The model under review builds one solid part; all positions refer to its coordinate system, in mm. A direction names the side the tool comes from. Round coordinates to 2 decimals unless told otherwise and drop trailing zeros. Order: outer loops, then holes, each group sorted by start corner. A loop starts at its lowest first (then second) coordinate and runs counter-clockwise, first axis right, second up. Notation, with made-up numbers: M 63,-20 L 74,-20 A16 ccw 74,-3 Z; hole C 75.5,35 d6. An arc over 180 degrees is marked long. Answer as a JSON object with one key per item and string values. Group by question number.
1. Add section A-A on z = 23. State the section outline as (x, y) points (1 decimal), and give its area (3 significant figures).
2. Clearance check with flat-ended pins moving along their axes: P1, Ø1.9, axis at x = -7.5, z = 31, coming from the -Y side; P2, Ø0.7, axis at y = 7.5, z = 37.5, coming from the -X side; P3, Ø0.5, axis at x = 0, y = -8, coming from the +Z side. State where each tip first meets the part, or that it passes through.
3. Add section D-D on z = 3. State the section outline as (x, y) points.
4. To check wall thickness, follow probe 1 along Y at (x, z) = (0, 23.5); probe 2 along Z at (x, y) = (4.75, 1.25); probe 3 along Y at (x, z) = (-3.5, 21) (3 decimals). State the ranges of each line that lie inside material, in increasing order. Write a range as [from, to].
5. Mouldability with a two-part tool opening along Y and no side actions: class faces 1 (the face through (-8, 0, 25)), 2 (the face through (-0.5, -8, 35)) as released by +Y, released by -Y, zero draft, split by the parting line, or undercut.
6. Machinability: for faces 3 (the face through (8, 0.5, 35)), 4 (the face through (0, -8, 25)), 5 (the face through (4.779, -4.876, 44.16)), which of the approach directions +Z, -Z, +X, -X, +Y, -Y give a long, thin tool a straight path to every point of the face, cutting with its end or side? Answer none if there is none.
7. Add section B-B on y = 0. State the section outline as (x, z) points.
```python
from build123d import *

# Parameters (mm, degrees)
SKETCH1_R           = 9
BOSS_EXTRUDE1_DEPTH = 45
SKETCH2_R           = 6.6675
CUT_EXTRUDE1_DEPTH  = 40
CHAMFER1_SIZE       = 1
SKETCH3_W           = 22.613634382
SKETCH3_H           = 1
SKETCH3_W_2         = 1
SKETCH3_H_2         = 23.145081594
CUT_EXTRUDE2_DEPTH  = 20


with BuildPart() as part:
    # Sketch1 → Boss-Extrude1 (new body)
    with BuildSketch(Plane.XY):
        with Locations(Location((0, 0, 0), (0, 0, 180))):
            Circle(SKETCH1_R)
    extrude(amount=BOSS_EXTRUDE1_DEPTH)

    # Sketch2 → Cut-Extrude1 (cut)
    with BuildSketch(Plane.XY.offset(45)):
        Circle(SKETCH2_R)
    extrude(amount=-CUT_EXTRUDE1_DEPTH, mode=Mode.SUBTRACT)

    # Chamfer1
    chamfer1_edges = [part.edges().sort_by_distance(p)[0] for p in [
        (-6.6675, 0, 45),
    ]]
    chamfer(chamfer1_edges, length=CHAMFER1_SIZE)

    # Sketch3 → Cut-Extrude2 (cut)
    with BuildSketch(Plane.XY.offset(45)):
        Rectangle(SKETCH3_W, SKETCH3_H)
        Rectangle(SKETCH3_W_2, SKETCH3_H_2)
    extrude(amount=-CUT_EXTRUDE2_DEPTH, mode=Mode.SUBTRACT)


solid = part.part
```
Recorded:
{
 "1": {"outline": "C 0,0 d18; hole C 0,0 d13.3", "area": "115 mm²"},
 "2": {"P1": "stops at y = -6.17", "P2": "stops at x = -5.47", "P3": "stops at z = 25"},
 "3": {"outline": "C 0,0 d18"},
 "4": {"probe 1": "y = [-9, -6.67], [6.67, 9]", "probe 2": "z = [0, 5]", "probe 3": "y = [-8.292, -5.675], [5.675, 8.292]"},
 "5": {"face 1": "undercut", "face 2": "zero draft"},
 "6": {"face 3": "+Z, +X, -X", "face 4": "+Z, +Y, -Y", "face 5": "+Z"},
 "7": {"outline": "M -9,0 L 9,0 L 9,25 L 6.67,25 L 6.67,5 L -6.67,5 L -6.67,25 L -9,25 Z"}
}
